from build123d import *

# Parameters (mm, degrees)
SKETCH1_R                      = 7.62
BOSS_EXTRUDE1_DEPTH            = 6.35
SKETCH2_R                      = 7.9375
CUT_EXTRUDE1_DEPTH             = 4.7625
SKETCH3_R                      = 7.9375
SKETCH3_R_2                    = 6.6675
BOSS_EXTRUDE2_DEPTH            = 4.75996
CHAMFER1_SIZE                  = 0.254
SKETCH4_R                      = 5.3975
SKETCH4_R_2                    = 4.7625
BOSS_EXTRUDE3_DEPTH            = 4.75996
CHAMFER2_SIZE                  = 0.254
SKETCH5_R                      = 6.6675
SKETCH5_R_2                    = 5.3975
BOSS_EXTRUDE4_DEPTH            = 4.2545
F_6_32_TAPPED_HOLE1_AT_2_COUNT = 2
F_6_32_TAPPED_HOLE1_AT_2_PITCH = 26.940768363


with BuildPart() as part:
    # Sketch1 → Boss-Extrude1 (new body)
    with BuildSketch(Plane(origin=(0, 0, 0), x_dir=(1, 0, 0), z_dir=(0, 1, 0))):
        with BuildLine():
            Line((-16.764, -16.51), (-7.62, -16.51))
            Line((-7.62, -16.51), (-7.62, -14.9479))
            ThreePointArc((-7.62, -14.9479), (-7.155032015, -13.825367985), (-6.0325, -13.3604))
            Line((-6.0325, -13.3604), (6.0325, -13.3604))
            ThreePointArc((6.0325, -13.3604), (7.155032015, -13.825367985), (7.62, -14.9479))
            Line((7.62, -14.9479), (7.62, -16.51))
            Line((7.62, -16.51), (16.764, -16.51))
            Line((16.764, -16.51), (16.764, -10.4267))
            Line((16.764, -10.4267), (15.1765, -10.4267))
            ThreePointArc((15.1765, -10.4267), (14.053967985, -9.961732015), (13.589, -8.8392))
            Line((13.589, -8.8392), (13.589, 8.8392))
            ThreePointArc((13.589, 8.8392), (14.053967985, 9.961732015), (15.1765, 10.4267))
            Line((15.1765, 10.4267), (16.764, 10.4267))
            Line((16.764, 10.4267), (16.764, 16.51))
            Line((16.764, 16.51), (7.62, 16.51))
            Line((7.62, 16.51), (7.62, 14.9479))
            ThreePointArc((7.62, 14.9479), (7.155032015, 13.825367985), (6.0325, 13.3604))
            Line((6.0325, 13.3604), (-6.0325, 13.3604))
            ThreePointArc((-6.0325, 13.3604), (-7.155032015, 13.825367985), (-7.62, 14.9479))
            Line((-7.62, 14.9479), (-7.62, 16.51))
            Line((-7.62, 16.51), (-16.764, 16.51))
            Line((-16.764, 16.51), (-16.764, 10.4267))
            Line((-16.764, 10.4267), (-15.1765, 10.4267))
            ThreePointArc((-15.1765, 10.4267), (-14.053967985, 9.961732015), (-13.589, 8.8392))
            Line((-13.589, 8.8392), (-13.589, -8.8392))
            ThreePointArc((-13.589, -8.8392), (-14.053967985, -9.961732015), (-15.1765, -10.4267))
            Line((-15.1765, -10.4267), (-16.764, -10.4267))
            Line((-16.764, -10.4267), (-16.764, -16.51))
        make_face()
        Circle(SKETCH1_R, mode=Mode.SUBTRACT)
    extrude(amount=BOSS_EXTRUDE1_DEPTH)

    # Sketch2 → Cut-Extrude1 (cut)
    with BuildSketch(Plane(origin=(0, 6.35, 0), x_dir=(1, 0, 0), z_dir=(0, 1, 0))):
        Circle(SKETCH2_R)
    extrude(amount=-CUT_EXTRUDE1_DEPTH, mode=Mode.SUBTRACT)

    # Sketch3 → Boss-Extrude2 (add)
    with BuildSketch(Plane(origin=(0, 1.5875, 0), x_dir=(-1, 0, 0), z_dir=(0, 1, 0))):
        Circle(SKETCH3_R)
        Circle(SKETCH3_R_2, mode=Mode.SUBTRACT)
    extrude(amount=BOSS_EXTRUDE2_DEPTH)

    # Chamfer1
    chamfer1_edges = [part.edges().sort_by_distance(p)[0] for p in [
        (6.6675, 1.5875, 0),
        (6.6675, 6.34746, 0),
    ]]
    chamfer(chamfer1_edges, length=CHAMFER1_SIZE)



with BuildPart() as body_2:
    # Sketch4 → Boss-Extrude3 (new body)
    with BuildSketch(Plane(origin=(0, 1.5875, 0), x_dir=(-1, 0, 0), z_dir=(0, 1, 0))):
        Circle(SKETCH4_R)
        Circle(SKETCH4_R_2, mode=Mode.SUBTRACT)
    extrude(amount=BOSS_EXTRUDE3_DEPTH)

    # Chamfer2
    chamfer2_edges = [body_2.edges().sort_by_distance(p)[0] for p in [
        (5.3975, 1.5875, 0),
        (5.3975, 6.34746, 0),
    ]]
    chamfer(chamfer2_edges, length=CHAMFER2_SIZE)


with BuildPart() as part_1:
    add(part.part)

    add(body_2.part)  # Boss-Extrude4 merges body 2
    # Sketch5 → Boss-Extrude4 (add)
    with BuildSketch(Plane(origin=(0, 6.09346, 0), x_dir=(-1, 0, 0), z_dir=(0, 1, 0))):
        Circle(SKETCH5_R)
        Circle(SKETCH5_R_2, mode=Mode.SUBTRACT)
    extrude(amount=-BOSS_EXTRUDE4_DEPTH)

    # Sketch8 → #6-32 Tapped Hole1 (revolve, cut)
    with BuildSketch(Plane(origin=(-16.764, 3.175, -13.470384182), x_dir=(0, 0, 1), z_dir=(0, 1, 0))):
        Polygon((0, 0), (0, 8.76289403), (1.35255, 7.9502), (1.35255, 7.0104), (1.7526, 7.0104), (1.7526, 0), align=None)
    f_6_32_tapped_hole1 = revolve(axis=Axis((-23.114, 3.175, -13.470384182), (1, 0, 0)), mode=Mode.SUBTRACT)

    # #6-32 Tapped Hole1 at 2: #6-32 Tapped Hole1 ×2
    with Locations(*[(0, 0, i * F_6_32_TAPPED_HOLE1_AT_2_PITCH) for i in range(1, F_6_32_TAPPED_HOLE1_AT_2_COUNT)]):
        add(f_6_32_tapped_hole1, mode=Mode.SUBTRACT)

    # Mirror1: #6-32 Tapped Hole1 across plane
    add(f_6_32_tapped_hole1.mirror(Plane(origin=(0, 0, 0), x_dir=(0, 0, 1), z_dir=(1, 0, 0))), mode=Mode.SUBTRACT)

    # Mirror1 copy 1 sketch → Mirror1 copy 1 (revolve, cut)
    with BuildSketch(Plane(origin=(16.764, 3.175, 13.470384182), x_dir=(0, 0, 1), z_dir=(0, 1, 0))):
        Polygon((0, 0), (0, -8.76289403), (1.35255, -7.9502), (1.35255, -7.0104), (1.7526, -7.0104), (1.7526, 0), align=None)
    revolve(axis=Axis((23.114, 3.175, 13.470384182), (1, 0, 0)), mode=Mode.SUBTRACT)


solid = part_1.part
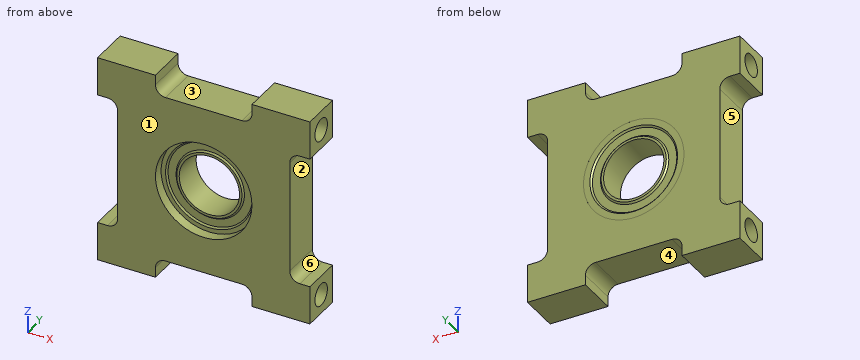
Can you work these out from the model? Positions are in its coordinate system, mm. Face numbers are marked on the shaded views. A direction names the side the tool comes from. Coordinates: 2 decimals unless noted, no trailing zeros. Loops run counter-clockwise (first coordinate to the right, second up) from the corner with the lowest first, then second, coordinate; pieces in that order, holes last. Notation, with made-up numbers: M 34,37.5 L 56,37.5 A23 ccw 56,56.5 Z; hole C 89.5,4 d4. An arc over 180 degrees is marked long. Return JSON: item names as keys, results as strings. Group by question number.
Item 1: On a 3-axis mill with a long thin cutter (end or side, diameter ignored), from which of +Z, -Z, +X, -X, +Y, -Y can I reach the whole of each face in a straight line? I mean the marked faces 4, 5 and 6. Say none if no direction works.
Item 2: If I drill on L1, parallel to Z at x = -12, y = 3; L2, parallel to X at y = 6.25, z = 0.5; L3, parallel to Z at x = 0, y = 0.85, over which ranges is the centre line in solid material (lowest first)? Write a range as from..to.
Item 3: Thinking about a two-plate mould opening in Z: for the marked faces 1, 2 and 3, which applies, released by +Z, released by -Z, zero draft, split by the parting line, or undercut?
Item 4: Imagine slicing it at A-A (x = -11.5). Please give me the cut outline in (y, z) (3 decimals), and give its area (3 significant figures).
Item 5: I'm going to push flat-ended pins straight in: pin 1 Ø1 at (x, y) = (-3.5, 2.5) entering from -Z; pin 2 Ø1.5 at (y, z) = (2, -9) entering from -X; pin 3 Ø1.6 at (y, z) = (3.18, 13.47) entering from -X. Where does each tip first touch, or does it pass through?
Verdict:
{
 "1": {"face 4": "-Z, +Y, -Y", "face 5": "-X, +Y, -Y", "face 6": "+X, +Y, -Y"},
 "2": {"L1": "z = -16.51..-15.21, -11.73..11.73, 15.21..16.51", "L2": "x = -13.59..-6.81, -5.22..-4.74, 4.74..5.22, 6.81..13.59", "L3": "z = -13.36..-7.62, 7.62..13.36"},
 "3": {"face 1": "zero draft", "face 2": "undercut", "face 3": "released by +Z"},
 "4": {"outline": "M 0,-16.51 L 6.35,-16.51 L 6.35,16.51 L 0,16.51 Z; hole C 3.175,-13.47 d3.505; hole C 3.175,13.47 d3.505", "area": "190 mm^2"},
 "5": {"pin 1": "stops at z = -13.36", "pin 2": "stops at x = -13.88", "pin 3": "stops at x = -8.48"}
}
